from build123d import *

# Parameters (mm, degrees)
BASE_EXTRUSION_DEPTH                 = 15.5875
BASE_EXTRUSION_DEPTH_BACK            = 88.9
PICKER_CLEARANCE_DEPTH               = 98.425
SKETCH3_W                            = 6.35
SKETCH3_H                            = 12.7
CLOTHES_LINE_NOTCH_DEPTH             = 237.446920576
TAB_TO_TOP_PLATE_DEPTH               = 6.35
TOP_PLATE_TABS_COUNT                 = 3
TOP_PLATE_TABS_PITCH                 = 38.1
SKETCH5_W                            = 6.35
SKETCH5_H                            = 25.408256086
BASE_PLATE_TAB_DEPTH                 = 6.35
BASE_PLATE_TAB_HOLES_COUNT           = 3
BASE_PLATE_TAB_HOLES_PITCH           = 38.1
SKETCH8_W                            = 12.7
SKETCH8_H                            = 6.35
BREAK_BEAM_DEPTH                     = 6.35
BREAK_BEAM_HOLES_COUNT               = 2
BREAK_BEAM_HOLES_PITCH               = 19.05
SKETCH10_R                           = 2.0955
CLOTHES_LINE_HOLE_DEPTH              = 239.906883011
CHASSIS_TOP_PLATE_T_SLOT_HOTES_DEPTH = 239.906883011
SKETCH12_R                           = 2.0955
CHASSIS_BASE_PLATE_HOLES_DEPTH       = 239.906883011
V_FUNNEL_CORNER_FILLET_R             = 7.62
BOSS_EXTRUDE1_DEPTH                  = 6.35
SKETCH14_W                           = 6.35
SKETCH14_H                           = 15.875
CUT_EXTRUDE1_DEPTH                   = 239.906883011
SKETCH16_W                           = 36.945833334
SKETCH16_H                           = 6.35
BOSS_EXTRUDE2_DEPTH                  = 6.35
SKETCH18_W                           = 29.464
SKETCH18_H                           = 8.4328
CUT_EXTRUDE2_DEPTH                   = 239.906883011
SKETCH19_W                           = 12.7
SKETCH19_H                           = 6.35
CUT_EXTRUDE3_DEPTH                   = 239.906883011
SKETCH22_W                           = 5.72
SKETCH22_H                           = 4.4
CUT_EXTRUDE6_DEPTH                   = 239.906883011


with BuildPart() as part:
    # Sketch1 → Base Extrusion (new, two sides: drawn at the far end of the back side and taken through both)
    with BuildSketch(Plane.XY.offset(-BASE_EXTRUSION_DEPTH_BACK)):
        Polygon((-4.490128061, -21.950964887), (0, -26.441092948), (-139.443807584, -165.884900532), (-143.933935645, -161.394772471), align=None)
    extrude(amount=BASE_EXTRUSION_DEPTH + BASE_EXTRUSION_DEPTH_BACK)

    # Sketch2 → Picker Clearance (cut)
    with BuildSketch(Plane(origin=(0, 0, -88.9), x_dir=(-1, 0, 0), z_dir=(0, 0, -1))):
        Polygon((12.347852166, -38.788945114), (16.837980227, -34.298817054), (28.063300378, -45.524137205), (23.573172318, -50.014265265), align=None)
    extrude(amount=-PICKER_CLEARANCE_DEPTH, mode=Mode.SUBTRACT)

    # Sketch3 → Clothes Line Notch (cut, through all)
    with BuildSketch(Plane(origin=(13.220546474, -13.220546474, 0), x_dir=(0, 0, -1), z_dir=(0.7071067811865477, -0.7071067811865474, 0))):
        with Locations((51.0875, -209.55)):
            Rectangle(SKETCH3_W, SKETCH3_H)
    extrude(amount=-CLOTHES_LINE_NOTCH_DEPTH, mode=Mode.SUBTRACT)

    # Sketch4 → Tab to Top Plate (add)
    with BuildSketch(Plane(origin=(0, 0, -88.9), x_dir=(-1, 0, 0), z_dir=(0, 0, -1))):
        Polygon((123.615619379, -150.056712327), (128.10574744, -145.566584266), (110.145235198, -127.606072024), (105.655107137, -132.096200085), align=None)
    tab_to_top_plate = extrude(amount=TAB_TO_TOP_PLATE_DEPTH)

    # Top Plate Tabs: Tab to Top Plate ×3
    with Locations(*[Vector(0.7071067811865476, 0.7071067811865476, 0) * (i * TOP_PLATE_TABS_PITCH) for i in range(1, TOP_PLATE_TABS_COUNT)]):
        add(tab_to_top_plate)

    # Sketch5 → Base Plate Tab (cut)
    with BuildSketch(Plane(origin=(8.730418413, -8.730418413, 0), x_dir=(0, 0, 1), z_dir=(-0.7071067811865477, 0.7071067811865475, 0))):
        with Locations((-3.175, -177.442548082)):
            Rectangle(SKETCH5_W, SKETCH5_H)
    base_plate_tab = extrude(amount=-BASE_PLATE_TAB_DEPTH, mode=Mode.SUBTRACT)

    # Base Plate Tab holes: Base Plate Tab ×3
    with Locations(*[Vector(0.7071067811865474, 0.7071067811865477, 0) * (i * BASE_PLATE_TAB_HOLES_PITCH) for i in range(1, BASE_PLATE_TAB_HOLES_COUNT)]):
        add(base_plate_tab, mode=Mode.SUBTRACT)

    # Sketch8 → Break Beam (cut)
    with BuildSketch(Plane(origin=(8.730418413, -8.730418413, 0), x_dir=(0, 0, 1), z_dir=(-0.7071067811865477, 0.7071067811865475, 0))):
        with Locations((-12.7, -206.375)):
            Rectangle(SKETCH8_W, SKETCH8_H)
    break_beam = extrude(amount=-BREAK_BEAM_DEPTH, mode=Mode.SUBTRACT)

    # Break Beam Holes: Break Beam ×2
    with Locations(*[(0, 0, -i * BREAK_BEAM_HOLES_PITCH) for i in range(1, BREAK_BEAM_HOLES_COUNT)]):
        add(break_beam, mode=Mode.SUBTRACT)

    # Sketch10 → Clothes Line Hole (cut, through all)
    with BuildSketch(Plane(origin=(13.220546474, -13.220546474, 0), x_dir=(0, 0, -1), z_dir=(0.7071067811865477, -0.7071067811865474, 0))):
        with Locations(Location((51.0875, -190.135614919, 0), (0, 0, 90))):
            Circle(SKETCH10_R)
    extrude(amount=-CLOTHES_LINE_HOLE_DEPTH, mode=Mode.SUBTRACT)

    # Sketch11 → Chassis top Plate T Slot Hotes (cut, through all)
    with BuildSketch(Plane(origin=(8.730418413, -8.730418413, 0), x_dir=(0.7071067811865475, 0.7071067811865477, 0), z_dir=(-0.7071067811865477, 0.7071067811865475, 0))):
        Polygon((-159.631961573, 88.9), (-163.899161573, 88.9), (-163.899161573, 80.137), (-166.210561573, 80.137), (-166.210561573, 76.962), (-163.899161573, 76.962), (-163.899161573, 73.66), (-159.631961573, 73.66), (-159.631961573, 76.962), (-157.320561573, 76.962), (-157.320561573, 80.137), (-159.631961573, 80.137), align=None)
        Polygon((-69.841268849, 88.9), (-74.108468849, 88.9), (-74.108468849, 80.137), (-76.419868849, 80.137), (-76.419868849, 76.962), (-74.108468849, 76.962), (-74.108468849, 73.66), (-69.841268849, 73.66), (-69.841268849, 76.962), (-67.529868849, 76.962), (-67.529868849, 80.137), (-69.841268849, 80.137), align=None)
        Polygon((-25.294326125, 88.9), (-29.561526125, 88.9), (-29.561526125, 80.137), (-31.872926125, 80.137), (-31.872926125, 76.962), (-29.561526125, 76.962), (-29.561526125, 73.66), (-25.294326125, 73.66), (-25.294326125, 76.962), (-22.982926125, 76.962), (-22.982926125, 80.137), (-25.294326125, 80.137), align=None)
    extrude(amount=-CHASSIS_TOP_PLATE_T_SLOT_HOTES_DEPTH, mode=Mode.SUBTRACT)

    # Sketch12 → Chassis Base Plate Holes (cut, through all)
    with BuildSketch(Plane(origin=(8.730418413, -8.730418413, 0), x_dir=(0.7071067811865475, 0.7071067811865477, 0), z_dir=(-0.7071067811865477, 0.7071067811865475, 0))):
        with Locations(Location((-202.846676125, 3.175, 0), (0, 0, 180))):
            Circle(SKETCH12_R)
        with Locations(Location((-70.290426125, 3.175, 0), (0, 0, 180))):
            Circle(SKETCH12_R)
        with Locations(Location((-27.427926125, 3.175, 0), (0, 0, 180))):
            Circle(SKETCH12_R)
    extrude(amount=-CHASSIS_BASE_PLATE_HOLES_DEPTH, mode=Mode.SUBTRACT)

    # V Funnel Corner Fillet
    v_funnel_corner_fillet_edges = [part.edges().sort_by_distance(p)[0] for p in [
        (-141.688871615, -163.639836502, 15.5875),
    ]]
    fillet(v_funnel_corner_fillet_edges, radius=V_FUNNEL_CORNER_FILLET_R)

    # Sketch13 → Boss-Extrude1 (add)
    with BuildSketch(Plane(origin=(8.730418413, -8.730418413, 0), x_dir=(0, 0, 1), z_dir=(-0.7071067811865477, 0.7071067811865475, 0))):
        Polygon((15.5875, -56.796676125), (15.5875, -31.396676125), (15.5875, -18.696676125), (21.9375, -18.696676125), (21.9375, -31.396676125), (21.9375, -56.796676125), (15.5875, -69.227964479), align=None)
    extrude(amount=-BOSS_EXTRUDE1_DEPTH)

    # Sketch14 → Cut-Extrude1 (cut, through all)
    with BuildSketch(Plane(origin=(8.730418413, -8.730418413, 0), x_dir=(0, 0, 1), z_dir=(-0.7071067811865477, 0.7071067811865475, 0))):
        with Locations((12.7, -44.096676125)):
            Rectangle(SKETCH14_W, SKETCH14_H)
    extrude(amount=-CUT_EXTRUDE1_DEPTH, mode=Mode.SUBTRACT)

    # Sketch16 → Boss-Extrude2 (add)
    with BuildSketch(Plane(origin=(-13.220546474, -13.220546474, 0), x_dir=(0, 0, -1), z_dir=(0.7071067811865519, 0.7071067811865431, 0))):
        with Locations((33.48125, -15.521676125)):
            Rectangle(SKETCH16_W, SKETCH16_H)
    extrude(amount=BOSS_EXTRUDE2_DEPTH)

    # Sketch18 → Cut-Extrude2 (cut, through all)
    with BuildSketch(Plane(origin=(8.730418413, -8.730418413, 0), x_dir=(0.7071067811865475, 0.7071067811865477, 0), z_dir=(-0.7071067811865477, 0.7071067811865475, 0))):
        with Locations((-194.818, 78.3336)):
            Rectangle(SKETCH18_W, SKETCH18_H)
    extrude(amount=-CUT_EXTRUDE2_DEPTH, mode=Mode.SUBTRACT)

    # Sketch19 → Cut-Extrude3 (cut, through all)
    with BuildSketch(Plane(origin=(8.730418413, -8.730418413, 0), x_dir=(0.7071067811865475, 0.7071067811865477, 0), z_dir=(-0.7071067811865477, 0.7071067811865475, 0))):
        with Locations((-18.696676125, 16.891)):
            Rectangle(SKETCH19_W, SKETCH19_H)
    extrude(amount=-CUT_EXTRUDE3_DEPTH, mode=Mode.SUBTRACT)

    # Sketch22 → Cut-Extrude6 (cut, through all)
    with BuildSketch(Plane(origin=(13.220546474, -13.220546474, 0), x_dir=(0, 0, -1), z_dir=(0.7071067811865475, -0.7071067811865476, 0))):
        with Locations((-6.3775, -27.246676125)):
            Rectangle(SKETCH22_W, SKETCH22_H)
    extrude(amount=-CUT_EXTRUDE6_DEPTH, mode=Mode.SUBTRACT)


solid = part.part
Geometry check sheet. Reference: the model listing, model coordinates, mm. A direction names the side the tool comes from. Coordinates: 2 decimals unless noted, no trailing zeros. Order: outer loops, then holes, each group sorted by start corner. A loop starts at its lowest first (then second) coordinate and runs counter-clockwise, first axis right, second up. Notation, with made-up numbers: (13, 82.5) - (27, 82.5) arc R10 cw to (27, 92.5) - close; hole circle Ø1 at (54, 0.25). An arc over 180 degrees is marked (long way). One line per item, written item: value.
(1) Sectioned sample at D-D (y = -108). Enter the section's corners in (x, z).
Data:
outline: (-90.54, -95.25) - (-81.56, -95.25) - (-81.56, -6.35) - (-90.54, -6.35) - close; (-90.54, 0) - (-81.56, 0) - (-81.56, 15.59) - (-90.54, 15.59) - close
(2) Depth check by flat-ended pin: pin 1 Ø8.5 at (x, y) = (-46.5, -68.5) entering from -Z; pin 2 Ø3 at (y, z) = (-80, -72) entering from -X; pin 3 Ø3 at (x, z) = (-114, -7.5) entering from +Y; pin 4 Ø8 at (x, y) = (-99, -122.5) entering from -Z. Enter the tip coordinate at first touch or a pass-through.
Data:
pin 1: stops at z = -88.9
pin 2: stops at x = -64.04
pin 3: stops at y = -129.96
pin 4: stops at z = -95.25
(3) Release check for a two-part mould opening along Z. For faces 1 (the face through (-135, -157, -25.4)), 2 (the face through (-76, -98, -88.9)), 3 (the face through (-2.28, -24.16, 3.86)) record: +Z half, -Z half, draft (parallel to the pull), parting line (faces both ways), or undercut.
Data:
face 1: undercut
face 2: -Z half
face 3: draft
(4) Sectioned sample at B-B (z = -61). Enter the section's corners in (x, y), and give its area (3 significant figures).
Data:
outline: (-143.93, -161.39) - (-139.44, -165.88) - (-23.57, -50.01) - (-28.06, -45.52) - close; (-16.84, -34.3) - (-12.35, -38.79) - (0, -26.44) - (-4.49, -21.95) - close
area: 1,150 mm^2
(5) Access from +Z, -Z, +X, -X, +Y, -Y to the whole of each face (thin tool, end or side, straight path). Record for faces 4 (the face through (-36.8, -58.7, -78.5)), 5 (the face through (-104.95, -126.84, -75.33)), 6 (the face through (-123.51, -145.4, -3.22)).
Data:
face 4: -X, -Y
face 5: -Z
face 6: +X, +Y
(6) Sectioned sample at A-A (z = -85). Enter the section's corners in (x, y), and give its area (3 significant figures).
Data:
outline: (-143.93, -161.39) - (-139.44, -165.88) - (-102.67, -129.11) - (-107.16, -124.62) - close; (-104.15, -121.61) - (-99.66, -126.1) - (-39.18, -65.62) - (-43.67, -61.13) - close; (-40.65, -58.12) - (-36.16, -62.61) - (-23.57, -50.01) - (-28.06, -45.52) - close; (-16.84, -34.3) - (-12.35, -38.79) - (-7.68, -34.12) - (-12.17, -29.63) - close; (-9.16, -26.62) - (-4.67, -31.11) - (0, -26.44) - (-4.49, -21.95) - close
area: 1,070 mm^2
(7) Sectioned sample at C-C (z = -17). Enter the section's corners in (x, y).
Data:
outline: (-143.93, -161.39) - (-139.44, -165.88) - (-134.95, -161.39) - (-139.44, -156.9) - close; (-134.95, -152.41) - (-130.46, -156.9) - (-23.57, -50.01) - (-28.06, -45.52) - close; (-16.84, -34.3) - (-12.35, -38.79) - (-4.49, -30.93) - (-8.98, -26.44) - close
(8) Thickness scan on probe 1 along Y at (x, z) = (-117.5, -44); probe 2 along Z at (x, y) = (-39, -60); probe 3 along X at (y, z) = (-105.5, 8.5). Record the ranges inside material, lowest first. Write a range as from..to.
Data:
probe 1: y = -143.94..-134.96
probe 2: z = -73.66..-5.25, -1.1..15.59
probe 3: x = -88.04..-79.06
